Build history of the part. All positions in model axes, mm. Coordinates: 2 decimals unless noted, no trailing zeros. Loops run counter-clockwise (first coordinate to the right, second up) from the corner with the lowest first, then second, coordinate; pieces in that order, holes last.
(1) Slice it at A-A (x = 169). Give the cut face in (y, z).
(2) Slice it at C-C (y = -181). Give the cut face in (x, z).
(3) Flat gauge pin, fed straight in: P1, Ø3, axis at x = 9, y = -29, coming from the +Z side. Where does the tip first touch, or does it go through?
(4) Slice it at B-B (z = 0.75). Give the number of separate pieces and of enclosed holes in the cut face, and give its area (3 significant figures).
(5) Wall check: L1, parallel to X at y = -189, z = 1.3; L2, parallel to Y at x = 36, z = 1.3; L3, parallel to Y at x = 169, z = 0.85. Give the ranges that are in metal, low to high.
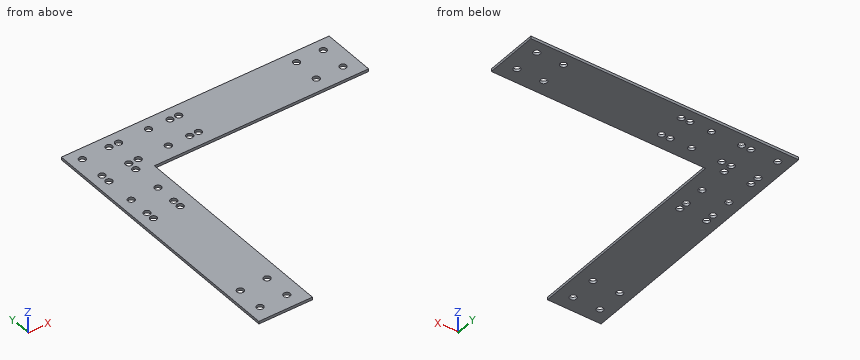
from build123d import *

# Parameters (mm, degrees)
F0_R     = 2.5
F1_DEPTH = 2


with BuildPart() as f1:
    # F0 (on Top) → F1 (new body)
    with BuildSketch(Plane.XY):
        with BuildLine():
            Line((40, 0), (0, 0))
            Line((0, 0), (0, -40))
            Line((0, -40), (9, -40))
            Line((9, -40), (9, -38.5))
            ThreePointArc((9, -38.5), (7.232233047, -34.232233047), (11.5, -36))
            Line((11.5, -36), (26.5, -36))
            ThreePointArc((26.5, -36), (27.232233047, -34.232233047), (29, -33.5))
            Line((29, -33.5), (29, -31.5))
            ThreePointArc((29, -31.5), (27.232233047, -27.232233047), (31.5, -29))
            Line((31.5, -29), (33.5, -29))
            ThreePointArc((33.5, -29), (34.232233047, -27.232233047), (36, -26.5))
            Line((36, -26.5), (36, -11.5))
            ThreePointArc((36, -11.5), (34.232233047, -7.232233047), (38.5, -9))
            Line((38.5, -9), (40, -9))
            Line((40, -9), (40, 0))
        make_face()
        with Locations((9, -29)):
            Circle(F0_R, mode=Mode.SUBTRACT)
        with Locations((9, -9)):
            Circle(F0_R, mode=Mode.SUBTRACT)
        with Locations((29, -9)):
            Circle(F0_R, mode=Mode.SUBTRACT)
        with BuildLine():
            Line((200, 0), (40, 0))
            Line((40, 0), (40, -9))
            Line((40, -9), (56, -9))
            ThreePointArc((56, -9), (58.5, -6.5), (61, -9))
            Line((61, -9), (72, -9))
            ThreePointArc((72, -9), (74.5, -6.5), (77, -9))
            Line((77, -9), (78.5, -9))
            ThreePointArc((78.5, -9), (81, -6.5), (83.5, -9))
            ThreePointArc((83.5, -9), (82.767766953, -10.767766953), (81, -11.5))
            Line((81, -11.5), (81, -26.5))
            ThreePointArc((81, -26.5), (82.767766953, -27.232233047), (83.5, -29))
            ThreePointArc((83.5, -29), (81, -31.5), (78.5, -29))
            Line((78.5, -29), (77, -29))
            ThreePointArc((77, -29), (74.5, -31.5), (72, -29))
            Line((72, -29), (61, -29))
            ThreePointArc((61, -29), (58.5, -31.5), (56, -29))
            Line((56, -29), (40, -29))
            Line((40, -29), (40, -40))
            Line((40, -40), (200, -40))
            Line((200, -40), (200, 0))
        make_face()
        with Locations((169, -29)):
            Circle(F0_R, mode=Mode.SUBTRACT)
        with Locations((189, -29)):
            Circle(F0_R, mode=Mode.SUBTRACT)
        with Locations((169, -9)):
            Circle(F0_R, mode=Mode.SUBTRACT)
        with Locations((189, -9)):
            Circle(F0_R, mode=Mode.SUBTRACT)
        with BuildLine():
            Line((9, -40), (0, -40))
            Line((0, -40), (0, -200))
            Line((0, -200), (40, -200))
            Line((40, -200), (40, -40))
            Line((40, -40), (29, -40))
            Line((29, -40), (29, -56))
            ThreePointArc((29, -56), (30.767766953, -56.732233047), (31.5, -58.5))
            ThreePointArc((31.5, -58.5), (30.767766953, -60.267766953), (29, -61))
            Line((29, -61), (29, -72))
            ThreePointArc((29, -72), (30.767766953, -72.732233047), (31.5, -74.5))
            ThreePointArc((31.5, -74.5), (30.767766953, -76.267766953), (29, -77))
            Line((29, -77), (29, -78.5))
            ThreePointArc((29, -78.5), (30.767766953, -79.232233047), (31.5, -81))
            ThreePointArc((31.5, -81), (29, -83.5), (26.5, -81))
            Line((26.5, -81), (11.5, -81))
            ThreePointArc((11.5, -81), (7.232233047, -82.767766953), (9, -78.5))
            Line((9, -78.5), (9, -77))
            ThreePointArc((9, -77), (6.5, -74.5), (9, -72))
            Line((9, -72), (9, -61))
            ThreePointArc((9, -61), (6.5, -58.5), (9, -56))
            Line((9, -56), (9, -40))
        make_face()
        with Locations((9, -189)):
            Circle(F0_R, mode=Mode.SUBTRACT)
        with Locations((29, -189)):
            Circle(F0_R, mode=Mode.SUBTRACT)
        with Locations((9, -169)):
            Circle(F0_R, mode=Mode.SUBTRACT)
        with Locations((29, -169)):
            Circle(F0_R, mode=Mode.SUBTRACT)
        with BuildLine():
            Line((40, -40), (40, -29))
            Line((40, -29), (38.5, -29))
            ThreePointArc((38.5, -29), (36, -31.5), (33.5, -29))
            Line((33.5, -29), (31.5, -29))
            ThreePointArc((31.5, -29), (30.767766953, -30.767766953), (29, -31.5))
            Line((29, -31.5), (29, -33.5))
            ThreePointArc((29, -33.5), (30.767766953, -34.232233047), (31.5, -36))
            ThreePointArc((31.5, -36), (30.767766953, -37.767766953), (29, -38.5))
            Line((29, -38.5), (29, -40))
            Line((29, -40), (40, -40))
        make_face()
        with BuildLine():
            Line((40, -29), (40, -9))
            Line((40, -9), (38.5, -9))
            ThreePointArc((38.5, -9), (37.767766953, -10.767766953), (36, -11.5))
            Line((36, -11.5), (36, -26.5))
            ThreePointArc((36, -26.5), (37.767766953, -27.232233047), (38.5, -29))
            Line((38.5, -29), (40, -29))
        make_face()
        with BuildLine():
            Line((56, -9), (40, -9))
            Line((40, -9), (40, -29))
            Line((40, -29), (56, -29))
            ThreePointArc((56, -29), (56.732233047, -27.232233047), (58.5, -26.5))
            Line((58.5, -26.5), (58.5, -11.5))
            ThreePointArc((58.5, -11.5), (56.732233047, -10.767766953), (56, -9))
        make_face()
        with BuildLine():
            Line((78.5, -9), (77, -9))
            ThreePointArc((77, -9), (76.267766953, -10.767766953), (74.5, -11.5))
            Line((74.5, -11.5), (74.5, -26.5))
            ThreePointArc((74.5, -26.5), (76.267766953, -27.232233047), (77, -29))
            Line((77, -29), (78.5, -29))
            ThreePointArc((78.5, -29), (79.232233047, -27.232233047), (81, -26.5))
            Line((81, -26.5), (81, -11.5))
            ThreePointArc((81, -11.5), (79.232233047, -10.767766953), (78.5, -9))
        make_face()
        with BuildLine():
            Line((72, -9), (61, -9))
            ThreePointArc((61, -9), (60.267766953, -10.767766953), (58.5, -11.5))
            Line((58.5, -11.5), (58.5, -26.5))
            ThreePointArc((58.5, -26.5), (60.267766953, -27.232233047), (61, -29))
            Line((61, -29), (72, -29))
            ThreePointArc((72, -29), (72.732233047, -27.232233047), (74.5, -26.5))
            Line((74.5, -26.5), (74.5, -11.5))
            ThreePointArc((74.5, -11.5), (72.732233047, -10.767766953), (72, -9))
        make_face()
        with BuildLine():
            Line((26.5, -74.5), (11.5, -74.5))
            ThreePointArc((11.5, -74.5), (10.767766953, -76.267766953), (9, -77))
            Line((9, -77), (9, -78.5))
            ThreePointArc((9, -78.5), (10.767766953, -79.232233047), (11.5, -81))
            Line((11.5, -81), (26.5, -81))
            ThreePointArc((26.5, -81), (27.232233047, -79.232233047), (29, -78.5))
            Line((29, -78.5), (29, -77))
            ThreePointArc((29, -77), (27.232233047, -76.267766953), (26.5, -74.5))
        make_face()
        with BuildLine():
            Line((26.5, -58.5), (11.5, -58.5))
            ThreePointArc((11.5, -58.5), (10.767766953, -60.267766953), (9, -61))
            Line((9, -61), (9, -72))
            ThreePointArc((9, -72), (10.767766953, -72.732233047), (11.5, -74.5))
            Line((11.5, -74.5), (26.5, -74.5))
            ThreePointArc((26.5, -74.5), (27.232233047, -72.732233047), (29, -72))
            Line((29, -72), (29, -61))
            ThreePointArc((29, -61), (27.232233047, -60.267766953), (26.5, -58.5))
        make_face()
        with BuildLine():
            Line((29, -40), (9, -40))
            Line((9, -40), (9, -56))
            ThreePointArc((9, -56), (10.767766953, -56.732233047), (11.5, -58.5))
            Line((11.5, -58.5), (26.5, -58.5))
            ThreePointArc((26.5, -58.5), (27.232233047, -56.732233047), (29, -56))
            Line((29, -56), (29, -40))
        make_face()
        with BuildLine():
            Line((9, -38.5), (9, -40))
            Line((9, -40), (29, -40))
            Line((29, -40), (29, -38.5))
            ThreePointArc((29, -38.5), (27.232233047, -37.767766953), (26.5, -36))
            Line((26.5, -36), (11.5, -36))
            ThreePointArc((11.5, -36), (10.767766953, -37.767766953), (9, -38.5))
        make_face()
    extrude(amount=F1_DEPTH)


solid = f1.part
Response values:
1. outline: (-40, 0) - (-31.5, 0) - (-31.5, 2) - (-40, 2) - close; (-26.5, 0) - (-11.5, 0) - (-11.5, 2) - (-26.5, 2) - close; (-6.5, 0) - (0, 0) - (0, 2) - (-6.5, 2) - close
2. outline: (0, 0) - (40, 0) - (40, 2) - (0, 2) - close
3. P1: passes through
4. separate pieces: 1
4. enclosed holes: 28
4. area: 13,900 mm2
5. L1: x = 0 to 6.5, 11.5 to 26.5, 31.5 to 40
5. L2: y = -200 to -31.5, -26.5 to -11.5, -6.5 to 0
5. L3: y = -40 to -31.5, -26.5 to -11.5, -6.5 to 0
